The listing builds one solid part. Answer for the finished solid, in the listing's coordinates (mm). A direction names the side the tool comes from. Coordinates: 2 decimals unless noted, no trailing zeros. Order: outer loops, then holes, each group sorted by start corner. A loop starts at its lowest first (then second) coordinate and runs counter-clockwise, first axis right, second up.
from build123d import *

# Parameters (mm, degrees)
SKETCH1_W           = 101.6
SKETCH1_H           = 88.9
BOSS_EXTRUDE1_DEPTH = 58.42
SKETCH2_W           = 91.44
SKETCH2_H           = 78.74
CUT_EXTRUDE1_DEPTH  = 55.88
SKETCH3_R           = 7.874
SKETCH3_R_2         = 2.032
CUT_EXTRUDE2_DEPTH  = 147.110726506
CUT_EXTRUDE3_DEPTH  = 147.110726506
SKETCH6_R           = 2.54
CUT_EXTRUDE4_DEPTH  = 144.639189638
SKETCH8_R           = 6.0325
CUT_EXTRUDE5_DEPTH  = 145.087642773
SKETCH9_W           = 96.52
SKETCH9_H           = 83.82
CUT_EXTRUDE6_DEPTH  = 2.54
SKETCH10_R          = 6.35
CUT_EXTRUDE7_DEPTH  = 145.087642773
BOSS_EXTRUDE2_DEPTH = 53.34
FILLET1_R           = 2.54
SKETCH13_R          = 1.524
CUT_EXTRUDE8_DEPTH  = 12.7


with BuildPart() as part:
    # Sketch1 → Boss-Extrude1 (new body)
    with BuildSketch(Plane(origin=(0, 0, 0), x_dir=(1, 0, 0), z_dir=(0, 1, 0))):
        with Locations((50.8, 44.45)):
            Rectangle(SKETCH1_W, SKETCH1_H)
    extrude(amount=BOSS_EXTRUDE1_DEPTH)

    # Sketch2 → Cut-Extrude1 (cut)
    with BuildSketch(Plane(origin=(0, 58.42, 0), x_dir=(1, 0, 0), z_dir=(0, 1, 0))):
        with Locations((50.8, 44.45)):
            Rectangle(SKETCH2_W, SKETCH2_H)
    extrude(amount=-CUT_EXTRUDE1_DEPTH, mode=Mode.SUBTRACT)

    # Sketch3 → Cut-Extrude2 (cut, through all)
    with BuildSketch(Plane(origin=(0, 2.54, 0), x_dir=(1, 0, 0), z_dir=(0, 1, 0))):
        with Locations(Location((14.605, 49.53, 0), (0, 0, 270))):
            Circle(SKETCH3_R)
        with Locations(Location((14.605, 65.278, 0), (0, 0, 270))):
            Circle(SKETCH3_R_2)
        with Locations(Location((14.605, 23.368, 0), (0, 0, 270))):
            Circle(SKETCH3_R_2)
    extrude(amount=-CUT_EXTRUDE2_DEPTH, mode=Mode.SUBTRACT)

    # Sketch5 → Cut-Extrude3 (cut, through all)
    with BuildSketch(Plane(origin=(0, 2.54, 0), x_dir=(1, 0, 0), z_dir=(0, 1, 0))):
        with BuildLine():
            ThreePointArc((49.279390438, 55.7784), (50.8, 33.02), (52.320609562, 55.7784))
            ThreePointArc((52.320609562, 55.7784), (50.8, 57.404), (49.279390438, 55.7784))
        make_face()
    extrude(amount=-CUT_EXTRUDE3_DEPTH, mode=Mode.SUBTRACT)

    # Sketch6 → Cut-Extrude4 (cut, through all)
    with BuildSketch(Plane.ZY.offset(-96.52)):
        with Locations((-17.526, 24.765)):
            Circle(SKETCH6_R)
        with Locations((-66.294, 24.765)):
            Circle(SKETCH6_R)
    extrude(amount=-CUT_EXTRUDE4_DEPTH, mode=Mode.SUBTRACT)

    # Sketch8 → Cut-Extrude5 (cut, through all)
    with BuildSketch(Plane(origin=(0, 0, -5.08), x_dir=(-1, 0, 0), z_dir=(0, 0, -1))):
        with Locations((-41.91, 20.32)):
            Circle(SKETCH8_R)
        with Locations((-59.69, 20.32)):
            Circle(SKETCH8_R)
    extrude(amount=-CUT_EXTRUDE5_DEPTH, mode=Mode.SUBTRACT)

    # Sketch9 → Cut-Extrude6 (cut)
    with BuildSketch(Plane(origin=(0, 58.42, 0), x_dir=(1, 0, 0), z_dir=(0, 1, 0))):
        with Locations((50.8, 44.45)):
            Rectangle(SKETCH9_W, SKETCH9_H)
    extrude(amount=-CUT_EXTRUDE6_DEPTH, mode=Mode.SUBTRACT)

    # Sketch10 → Cut-Extrude7 (cut, through all)
    with BuildSketch(Plane(origin=(0, 0, -5.08), x_dir=(-1, 0, 0), z_dir=(0, 0, -1))):
        with Locations((-50.8, 40.64)):
            Circle(SKETCH10_R)
    extrude(amount=-CUT_EXTRUDE7_DEPTH, mode=Mode.SUBTRACT)

    # Sketch11 → Boss-Extrude2 (add)
    with BuildSketch(Plane(origin=(0, 2.54, 0), x_dir=(1, 0, 0), z_dir=(0, 1, 0))):
        with BuildLine():
            Line((10.16, 83.82), (5.08, 83.82))
            Line((5.08, 83.82), (5.08, 78.74))
            ThreePointArc((5.08, 78.74), (8.672102448, 80.227897552), (10.16, 83.82))
        make_face()
        with BuildLine():
            Line((5.08, 10.16), (5.08, 5.08))
            Line((5.08, 5.08), (10.16, 5.08))
            ThreePointArc((10.16, 5.08), (8.672102448, 8.672102448), (5.08, 10.16))
        make_face()
        with BuildLine():
            Line((96.52, 10.16), (96.52, 5.08))
            Line((96.52, 5.08), (91.44, 5.08))
            ThreePointArc((91.44, 5.08), (92.927897552, 8.672102448), (96.52, 10.16))
        make_face()
        with BuildLine():
            Line((96.52, 78.74), (96.52, 83.82))
            Line((96.52, 83.82), (91.44, 83.82))
            ThreePointArc((91.44, 83.82), (92.927897552, 80.227897552), (96.52, 78.74))
        make_face()
    extrude(amount=BOSS_EXTRUDE2_DEPTH)

    # Fillet1
    fillet1_edges = [part.edges().sort_by_distance(p)[0] for p in [
        (91.44, 29.21, -5.08),
        (96.52, 29.21, -10.16),
        (91.44, 29.21, -83.82),
        (96.52, 29.21, -78.74),
        (5.08, 29.21, -78.74),
        (10.16, 29.21, -83.82),
        (10.16, 29.21, -5.08),
        (5.08, 29.21, -10.16),
    ]]
    fillet(fillet1_edges, radius=FILLET1_R)

    # Sketch13 → Cut-Extrude8 (cut)
    with BuildSketch(Plane(origin=(0, 55.88, 0), x_dir=(1, 0, 0), z_dir=(0, 1, 0))):
        with Locations(Location((6.35, 82.55, 0), (0, 0, 270))):
            Circle(SKETCH13_R)
        with Locations(Location((95.25, 82.55, 0), (0, 0, 270))):
            Circle(SKETCH13_R)
        with Locations(Location((95.25, 6.35, 0), (0, 0, 270))):
            Circle(SKETCH13_R)
        with Locations(Location((6.35, 6.35, 0), (0, 0, 270))):
            Circle(SKETCH13_R)
    extrude(amount=-CUT_EXTRUDE8_DEPTH, mode=Mode.SUBTRACT)


solid = part.part
(1) Given pin 1 Ø11 at (x, y) = (41.91, 20.32) entering from +Z; pin 2 Ø14 at (x, z) = (14.605, -49.53) entering from +Y; pin 3 Ø8 at (x, z) = (28, -73) entering from -Y; pin 4 Ø12 at (x, z) = (68.5, -50.5) entering from +Y, each flat-ended and moving along its own axis, determine where each tip first touches the part or whether it passes through.
(2) A tool of negligible diameter and unlimited length cuts with its end or side. For faces 1 (the flat face through (101.6, 29, -44)), 2 (the cylindrical face through (5.56, 29.58, -78.12)), 3 (the cylindrical face through (56.45, 25.41, -2.58)), from which of +Z, -Z, +X, -X, +Y, -Y can it reach the whole face along a straight path? Write none if from no direction.
(3) Find section B-B on x = 41.91. Determine the outline of the cut face in (y, z), then the cut area to 3 significant figures.
(4) Find section D-D on y = 40.64. Determine the outline of the cut face in (x, z), then the cut area to 3 significant figures.
(5) The mould has two halves that part along Z. Classify faces 4 (the flat face through (50, 29, 0)), 5 (the flat face through (6, 43.18, -6)), 6 (the flat face through (99.06, 57, -44)), 7 (the flat face through (0, 29, -44)): pulls with the +Z half, pulls with the -Z half, needs draft (parallel to the pull), parting line crosses it, or undercut.
(6) Find the intervals of material crossed by probe 1 along X at (y, z) = (53, -45); probe 2 along Z at (x, y) = (15.5, 34.5); probe 3 along X at (y, z) = (1.65, -44.45), in increasing order.
(7) Find section A-A on y = 20.32. Determine the outline of the cut face in (x, z), then the cut area to 3 significant figures.
(8) Find section C-C on z = -47.5. Determine the outline of the cut face in (x, y), then the cut area to 3 significant figures.
Resolved:
1. pin 1: stops at z = -83.82
1. pin 2: passes through
1. pin 3: stops at y = 0
1. pin 4: stops at y = 2.54
2. face 1: +Z, -Z, +X, +Y, -Y
2. face 2: +Y
2. face 3: +Z
3. outline: (0, -88.9) - (58.42, -88.9) - (58.42, -86.36) - (55.88, -86.36) - (55.88, -83.82) - (2.54, -83.82) - (2.54, -51.63) - (0, -51.63) - close; (0, -37.27) - (2.54, -37.27) - (2.54, -5.08) - (14.29, -5.08) - (14.29, 0) - (0, 0) - close; (26.35, -5.08) - (55.88, -5.08) - (55.88, -2.54) - (58.42, -2.54) - (58.42, 0) - (26.35, 0) - close
3. area: 683 mm2
4. outline: (0, -88.9) - (101.6, -88.9) - (101.6, 0) - (57.15, 0) - (57.15, -5.08) - (89.34, -5.08) arc R2.54 cw to (91.73, -6.77) arc R5.08 ccw to (94.83, -9.87) arc R2.54 cw to (96.52, -12.26) - (96.52, -76.64) arc R2.54 cw to (94.83, -79.03) arc R5.08 ccw to (91.73, -82.13) arc R2.54 cw to (89.34, -83.82) - (12.26, -83.82) arc R2.54 cw to (9.87, -82.13) arc R5.08 ccw to (6.77, -79.03) arc R2.54 cw to (5.08, -76.64) - (5.08, -12.26) arc R2.54 cw to (6.77, -9.87) arc R5.08 ccw to (9.87, -6.77) arc R2.54 cw to (12.26, -5.08) - (44.45, -5.08) - (44.45, 0) - (0, 0) - close
4. area: 1,850 mm2
5. face 4: pulls with the +Z half
5. face 5: undercut
5. face 6: undercut
5. face 7: needs draft
6. probe 1: x = 0 to 5.08, 96.52 to 101.6
6. probe 2: z = -88.9 to -83.82, -5.08 to 0
6. probe 3: x = 0 to 8.59, 20.62 to 39.37, 62.23 to 101.6
7. outline: (0, -88.9) - (101.6, -88.9) - (101.6, 0) - (65.72, 0) - (65.72, -5.08) - (89.34, -5.08) arc R2.54 cw to (91.73, -6.77) arc R5.08 ccw to (94.83, -9.87) arc R2.54 cw to (96.52, -12.26) - (96.52, -76.64) arc R2.54 cw to (94.83, -79.03) arc R5.08 ccw to (91.73, -82.13) arc R2.54 cw to (89.34, -83.82) - (12.26, -83.82) arc R2.54 cw to (9.87, -82.13) arc R5.08 ccw to (6.77, -79.03) arc R2.54 cw to (5.08, -76.64) - (5.08, -12.26) arc R2.54 cw to (6.77, -9.87) arc R5.08 ccw to (9.87, -6.77) arc R2.54 cw to (12.26, -5.08) - (35.88, -5.08) - (35.88, 0) - (0, 0) - close; (47.94, -5.08) - (53.66, -5.08) - (53.66, 0) - (47.94, 0) - close
7. area: 1,800 mm2
8. outline: (0, 0) - (7, 0) - (7, 2.54) - (5.08, 2.54) - (5.08, 55.88) - (2.54, 55.88) - (2.54, 58.42) - (0, 58.42) - close; (22.21, 0) - (39.78, 0) - (39.78, 2.54) - (22.21, 2.54) - close; (61.82, 0) - (101.6, 0) - (101.6, 58.42) - (99.06, 58.42) - (99.06, 55.88) - (96.52, 55.88) - (96.52, 2.54) - (61.82, 2.54) - close
8. area: 718 mm2
